Autodesk Inventor part; units mm, degrees
ref_plane "YZ Plane" through (0, 0, 0) normal (1, 0, 0) x (0, 1, 0)
ref_plane "XZ Plane" through (0, 0, 0) normal (0, 1, 0) x (-1, 0, 0)
ref_plane "XY Plane" through (0, 0, 0) normal (0, 0, 1) x (1, 0, 0)
sketch "Sketch1" plane through (0, 0, 0) normal (0, 1, 0) x (-1, 0, 0)
  circle A0 centre (16.5875, 0) radius 2.5 construction
  circle A1 centre (-16.5875, 0) radius 2.5 construction
  line L0 (16.5875, 0) -> (-16.5875, 0) construction
  circle A2 centre (10.5875, 6) radius 2.1
  circle A3 centre (10.5875, -6) radius 2.1
  circle A4 centre (22.5875, -6) radius 2.1
  circle A5 centre (22.5875, 6) radius 2.1
  circle A6 centre (-22.5875, -6) radius 2.1
  circle A7 centre (-10.5875, -6) radius 2.1
  circle A8 centre (-10.5875, 6) radius 2.1
  circle A9 centre (-22.5875, 6) radius 2.1
  line L1 (29.3, 12.7) -> (-29.3, 12.7)
  line L2 (-29.3, 12.7) -> (-29.3, -12.7)
  line L3 (-29.3, -12.7) -> (29.3, -12.7)
  line L4 (29.3, -12.7) -> (29.3, 12.7)
  line L5 (29.3, 12.7) -> (-29.3, -12.7) construction
  line L6 (-29.3, 12.7) -> (29.3, -12.7) construction
  point P0 (0, 0)
  point P1 (0, 0)
  dimension "d0" = 5
  dimension "d1" = 5
  dimension "d2" = 33.175
  dimension "d3" = 4.2
  dimension "d4" = 6
  dimension "d5" = 6
  dimension "d8" = 360
  dimension "d10" = 4.2
  dimension "d11" = 6
  dimension "d12" = 6
  dimension "d15" = 360
  dimension "d17" = 58.6
  dimension "d18" = 25.4
extrude "Extrusion1" add sketch "Sketch1" along normal blind 3.175
chamfer "Chamfer1" distance 4 angle 45 4 edges at (-29.3, 1.5875, 12.7) (29.3, 1.5875, 12.7) (29.3, 1.5875, -12.7) (-29.3, 1.5875, -12.7)
properties part number "MotorMoutningTopConnectionPlate"
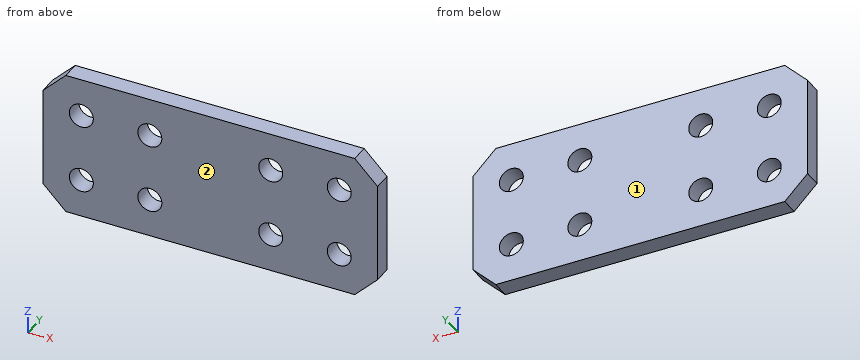
CAD build for the part. Positions are in the model's coordinates, mm. Face numbers are marked on the shaded views. Coordinates: 2 decimals unless noted, no trailing zeros. Write each loop counter-clockwise with the first axis right and the second up, starting at its lowest first coordinate (ties: lowest second). Pieces come first, ordered by that corner, then holes. Notation, with made-up numbers: M 46.5,21.25 L 83.5,21.25 A17 cw 83.5,45.25 Z; hole C 34,-0.5 d7. An arc over 180 degrees is marked long. Return JSON: item names as keys, results as strings.
Item 1: Slice it at D-D, the plane z = -6.75. Write the cut outline in (x, y) (3 decimals), and give its area (3 significant figures).
Findings below:
{"outline": "M -29.3,0 L -24.549,0 L -24.549,3.175 L -29.3,3.175 Z; M -20.626,0 L -12.549,0 L -12.549,3.175 L -20.626,3.175 Z; M -8.626,0 L 8.626,0 L 8.626,3.175 L -8.626,3.175 Z; M 12.549,0 L 20.626,0 L 20.626,3.175 L 12.549,3.175 Z; M 24.549,0 L 29.3,0 L 29.3,3.175 L 24.549,3.175 Z", "area": "136 mm2"}
Item 2: Drop a flat-ended pin along its axis: pin 1 Ø3.5 at (x, z) = (-10.59, -6) entering from -Y. Give the stop position or say it passes through.
Findings below:
{"pin 1": "passes through"}
Item 3: Slice it at C-C, the plane z = -9.5. Write the cut outline in (x, y) (3 decimals).
Findings below:
{"outline": "M -28.5,0 L 28.5,0 L 28.5,3.175 L -28.5,3.175 Z"}
Item 4: Slice it at B-B, the plane y = 0.6. State how many separate pieces and enclosed holes the cut face has, and give its area (3 significant figures).
Findings below:
{"separate pieces": "1", "enclosed holes": "8", "area": "1,350 mm2"}
Item 5: Two-plate mould, pull along Y, no slides. Class the marked faces 1 and 2: +Y half, -Y half, draft (parallel to the pull), parting line (faces both ways), or undercut.
Findings below:
{"face 1": "+Y half", "face 2": "-Y half"}
Item 6: Slice it at A-A, the plane z = 6. Write the cut outline in (x, y) (1 decimal).
Findings below:
{"outline": "M -29.3,0 L -24.7,0 L -24.7,3.2 L -29.3,3.2 Z; M -20.5,0 L -12.7,0 L -12.7,3.2 L -20.5,3.2 Z; M -8.5,0 L 8.5,0 L 8.5,3.2 L -8.5,3.2 Z; M 12.7,0 L 20.5,0 L 20.5,3.2 L 12.7,3.2 Z; M 24.7,0 L 29.3,0 L 29.3,3.2 L 24.7,3.2 Z"}
Item 7: Probe line 1 (Z direction, x = 12, y = 1.2); line 2 (X direction, y = 1.05, z = -5); line 3 (Z direction, x = 22, y = 2.75). List the from-to ranges inside material, lowest first. Write a range as from..to.
Findings below:
{"line 1": "z = -12.7..-7.55, -4.45..4.45, 7.55..12.7", "line 2": "x = -29.3..-24.43, -20.74..-12.43, -8.74..8.74, 12.43..20.74, 24.43..29.3", "line 3": "z = -12.7..-8.02, -3.98..3.98, 8.02..12.7"}
